```python
from build123d import *

# Parameters (mm, degrees)
SZKIC1_R                    = 20
DODANIE_WYCI_GNI_CIE1_DEPTH = 50
ZAOKR_GLENIE1_R             = 5
SZKIC2_R                    = 8
DODANIE_WYCI_GNI_CIE2_DEPTH = 50
SZKIC3_R                    = 6
DODANIE_WYCI_GNI_CIE3_DEPTH = 60


with BuildPart() as part:
    # Szkic1 → Dodanie-wyciągnięcie1 (new body)
    with BuildSketch(Plane.XY):
        Circle(SZKIC1_R)
    extrude(amount=DODANIE_WYCI_GNI_CIE1_DEPTH)

    # Zaokrąglenie1
    zaokr_glenie1_edges = [part.edges().sort_by_distance(p)[0] for p in [
        (-20, 0, 0),
        (-20, 0, 50),
    ]]
    fillet(zaokr_glenie1_edges, radius=ZAOKR_GLENIE1_R)

    # Szkic2 → Dodanie-wyciągnięcie2 (add)
    with BuildSketch(Plane.XY.offset(50)):
        Circle(SZKIC2_R)
    extrude(amount=DODANIE_WYCI_GNI_CIE2_DEPTH)

    # Szkic3 → Dodanie-wyciągnięcie3 (add)
    with BuildSketch(Plane(origin=(0, 0, 0), x_dir=(0, 0, -1), z_dir=(1, 0, 0))):
        with Locations((-19.389494998, 0)):
            Circle(SZKIC3_R)
    extrude(amount=DODANIE_WYCI_GNI_CIE3_DEPTH)


solid = part.part
```
Check sheet for the modelled part. Datum: model origin and axes. Units: mm. A direction names the side the tool comes from. Give positions to 0.01 mm unless a question says otherwise; leave off trailing zeros. Write each loop counter-clockwise with the first axis right and the second up, starting at its lowest first coordinate (ties: lowest second). Pieces come first, ordered by that corner, then holes.
Item 1: Scan lines: L1, parallel to Z at x = 28, y = 0; L2, parallel to X at y = -0.5, z = 11; L3, parallel to Z at x = 7, y = -9. Record each from-to range of solid material in increasing order.
Item 2: Access from +Z, -Z, +X, -X, +Y, -Y to the whole of each face (thin tool, end or side, straight path). Record for faces 1 (the face through (39.253, 0.264, 25.384)), 2 (the face through (-1.73, -7.81, 74.65)), 3 (the face through (0, 0, 100)).
Item 3: Gauge pin test, flat ends, axial feed: pin 1 (8 mm diameter, centred on x = 39, y = -6, fed in from +Z); pin 2 (10 mm diameter, centred on x = 14, z = 12, fed in from -Y); pin 3 (1 mm diameter, centred on y = 6.5, z = 52, fed in from -X). Record the tip position at first contact, or that the pin passes through.
Item 4: Cross-section at A-A (y = 0). Enter the section's corners in (x, z).
Item 5: Cross-section at D-D (x = 41.5). Enter the section's corners in (y, z).
Item 6: Cross-section at C-C (z = 29.5). Enter the section's corners in (x, y).
Item 7: Cross-section at B-B (x = 0). Enter the section's corners in (y, z), and give its area (3 significant figures).
Report:
1. L1: z = 13.39 to 25.39
1. L2: x = -19.99 to 19.99
1. L3: z = 0 to 50
2. face 1: +X
2. face 2: +Z
2. face 3: +Z, +X, -X, +Y, -Y
3. pin 1: stops at z = 25.05
3. pin 2: stops at y = -17.86
3. pin 3: stops at x = -5.29
4. outline: (-20, 5) arc R5 ccw to (-15, 0) - (15, 0) arc R5 ccw to (20, 5) - (20, 13.39) - (60, 13.39) - (60, 25.39) - (20, 25.39) - (20, 45) arc R5 ccw to (15, 50) - (8, 50) - (8, 100) - (-8, 100) - (-8, 50) - (-15, 50) arc R5 ccw to (-20, 45) - close
5. outline: circle Ø12 at (0, 19.39)
6. outline: circle Ø40 at (0, 0)
7. outline: (-20, 5) arc R5 ccw to (-15, 0) - (15, 0) arc R5 ccw to (20, 5) - (20, 45) arc R5 ccw to (15, 50) - (8, 50) - (8, 100) - (-8, 100) - (-8, 50) - (-15, 50) arc R5 ccw to (-20, 45) - close
7. area: 2,780 mm2
